Work out the finished part from the listing and answer in its coordinate system (mm). A direction names the side the tool comes from. Give positions to 0.01 mm unless a question says otherwise; leave off trailing zeros. Order: outer loops, then holes, each group sorted by start corner. A loop starts at its lowest first (then second) coordinate and runs counter-clockwise, first axis right, second up. Notation, with made-up numbers: M 86.5,-6 L 93.5,-6 A20 cw 93.5,10 Z; hole C 43.25,-25.5 d5. An arc over 180 degrees is marked long. One line per item, written item: value.
from build123d import *

# Parameters (mm, degrees)
BOSS_EXTRUDE1_DEPTH = 2
CHAMFER1_SIZE       = 12
SKETCH2_R           = 1.5
CUT_EXTRUDE1_DEPTH  = 10


with BuildPart() as part:
    # Sketch1 → Boss-Extrude1 (new body)
    with BuildSketch(Plane(origin=(0, 0, 0), x_dir=(1, 0, 0), z_dir=(0, 1, 0))):
        Polygon((-25.833763343, 95.703211573), (11.576236657, 95.703211573), (11.576236657, -6.301788427), (-25.833763343, -6.301788427), (-45.833763343, 13.698211573), (-45.833763343, 75.703211573), align=None)
        with BuildLine():
            Line((1.925471464, 43.200711573), (-28.074528536, 43.200711573))
            ThreePointArc((-28.074528536, 43.200711573), (-29.574528536, 44.700711573), (-28.074528536, 46.200711573))
            Line((-28.074528536, 46.200711573), (1.925471464, 46.200711573))
            ThreePointArc((1.925471464, 46.200711573), (3.425471464, 44.700711573), (1.925471464, 43.200711573))
        make_face(mode=Mode.SUBTRACT)
        with BuildLine():
            Line((1.925471464, 53.200711573), (-28.074528536, 53.200711573))
            ThreePointArc((-28.074528536, 53.200711573), (-29.574528536, 54.700711573), (-28.074528536, 56.200711573))
            Line((-28.074528536, 56.200711573), (1.925471464, 56.200711573))
            ThreePointArc((1.925471464, 56.200711573), (3.425471464, 54.700711573), (1.925471464, 53.200711573))
        make_face(mode=Mode.SUBTRACT)
        with BuildLine():
            Line((1.925471464, 63.200711573), (-28.074528536, 63.200711573))
            ThreePointArc((-28.074528536, 63.200711573), (-29.574528536, 64.700711573), (-28.074528536, 66.200711573))
            Line((-28.074528536, 66.200711573), (1.925471464, 66.200711573))
            ThreePointArc((1.925471464, 66.200711573), (3.425471464, 64.700711573), (1.925471464, 63.200711573))
        make_face(mode=Mode.SUBTRACT)
        with BuildLine():
            Line((1.925471464, 73.200711573), (-28.074528536, 73.200711573))
            ThreePointArc((-28.074528536, 73.200711573), (-29.574528536, 74.700711573), (-28.074528536, 76.200711573))
            Line((-28.074528536, 76.200711573), (1.925471464, 76.200711573))
            ThreePointArc((1.925471464, 76.200711573), (3.425471464, 74.700711573), (1.925471464, 73.200711573))
        make_face(mode=Mode.SUBTRACT)
        with BuildLine():
            Line((1.925471464, 83.200711573), (-28.074528536, 83.200711573))
            ThreePointArc((-28.074528536, 83.200711573), (-29.574528536, 84.700711573), (-28.074528536, 86.200711573))
            Line((-28.074528536, 86.200711573), (1.925471464, 86.200711573))
            ThreePointArc((1.925471464, 86.200711573), (3.425471464, 84.700711573), (1.925471464, 83.200711573))
        make_face(mode=Mode.SUBTRACT)
        with BuildLine():
            Line((1.925471464, 36.200711573), (-28.074528536, 36.200711573))
            ThreePointArc((-28.074528536, 36.200711573), (-29.574528536, 34.700711573), (-28.074528536, 33.200711573))
            Line((-28.074528536, 33.200711573), (1.925471464, 33.200711573))
            ThreePointArc((1.925471464, 33.200711573), (3.425471464, 34.700711573), (1.925471464, 36.200711573))
        make_face(mode=Mode.SUBTRACT)
        with BuildLine():
            Line((1.925471464, 26.200711573), (-28.074528536, 26.200711573))
            ThreePointArc((-28.074528536, 26.200711573), (-29.574528536, 24.700711573), (-28.074528536, 23.200711573))
            Line((-28.074528536, 23.200711573), (1.925471464, 23.200711573))
            ThreePointArc((1.925471464, 23.200711573), (3.425471464, 24.700711573), (1.925471464, 26.200711573))
        make_face(mode=Mode.SUBTRACT)
        with BuildLine():
            Line((1.925471464, 16.200711573), (-28.074528536, 16.200711573))
            ThreePointArc((-28.074528536, 16.200711573), (-29.574528536, 14.700711573), (-28.074528536, 13.200711573))
            Line((-28.074528536, 13.200711573), (1.925471464, 13.200711573))
            ThreePointArc((1.925471464, 13.200711573), (3.425471464, 14.700711573), (1.925471464, 16.200711573))
        make_face(mode=Mode.SUBTRACT)
        with BuildLine():
            Line((1.925471464, 6.200711573), (-28.074528536, 6.200711573))
            ThreePointArc((-28.074528536, 6.200711573), (-29.574528536, 4.700711573), (-28.074528536, 3.200711573))
            Line((-28.074528536, 3.200711573), (1.925471464, 3.200711573))
            ThreePointArc((1.925471464, 3.200711573), (3.425471464, 4.700711573), (1.925471464, 6.200711573))
        make_face(mode=Mode.SUBTRACT)
    extrude(amount=BOSS_EXTRUDE1_DEPTH)

    # Chamfer1
    chamfer1_edges = [part.edges().sort_by_distance(p)[0] for p in [
        (11.576236657, 1, -95.703211573),
        (11.576236657, 1, 6.301788427),
    ]]
    chamfer(chamfer1_edges, length=CHAMFER1_SIZE)

    # Sketch2 → Cut-Extrude1 (cut)
    with BuildSketch(Plane(origin=(0, 2, 0), x_dir=(1, 0, 0), z_dir=(0, 1, 0))):
        with Locations(Location((-4.838827122, 92.166588575, 0), (0, 0, 270))):
            Circle(SKETCH2_R)
        with Locations(Location((-41.371381926, 72.921675145, 0), (0, 0, 270))):
            Circle(SKETCH2_R)
        with Locations(Location((-41.371381926, 16.479748001, 0), (0, 0, 270))):
            Circle(SKETCH2_R)
        with Locations(Location((-4.838827122, -2.765165428, 0), (0, 0, 270))):
            Circle(SKETCH2_R)
    extrude(amount=-CUT_EXTRUDE1_DEPTH, mode=Mode.SUBTRACT)


solid = part.part
(1) Which of the six approach directions +Z, -Z, +X, -X, +Y, -Y give full straight-line access (tool end or side, diameter ignored) to faces 4 (the flat face through (-13, 1, 6.302)), 5 (the cylindrical face through (3.425, 0.986, -74.734))?
Findings:
face 4: +Z, +X, -X, +Y, -Y
face 5: +Y, -Y
(2) Determine the mould class of faces 1 (the flat face through (-13, 1, -66.201)), 2 (the flat face through (-17, 0, -57)), 3 (the flat face through (-17, 2, -57)) for opening direction Y: pulls with the +Y half, pulls with the -Y half, needs draft (parallel to the pull), parting line crosses it, or undercut.
Findings:
face 1: needs draft
face 2: pulls with the -Y half
face 3: pulls with the +Y half
(3) Find the intervals of material crossed by probe 1 along Z at (x, y) = (-40, 1.6); probe 2 along Z at (x, y) = (-41.5, 1.3); probe 3 along X at (y, z) = (0.4, -46), in increasing order. Write a range as from..to.
Findings:
probe 1: z = -81.54..-73.53, -72.31..-17.09, -15.87..-7.86
probe 2: z = -80.04..-74.42, -71.43..-17.97, -14.99..-9.36
probe 3: x = -45.83..-28.82, 2.68..11.58
(4) Section D-D, the plane z = -8.5 is taken. Give the vertices of the cut face in (x, y).
Findings:
outline: M -40.64,0 L 11.58,0 L 11.58,2 L -40.64,2 Z
(5) Given P1, Ø1, axis at x = -38.5, y = 0.5, coming from the -Z side, flat-ended and moving along its own axis, determine where the tip first touches the part or whether it passes through.
Findings:
P1: stops at z = -83.54
(6) Section B-B, the plane x = -17.5 is taken. Give the number of separate pieces and of enclosed holes in the cut face, then the cut area to 3 significant figures.
Findings:
separate pieces: 10
enclosed holes: 0
area: 150 mm^2
(7) Section A-A, the plane z = -65 is taken. Give the vertices of the cut face in (x, y), then the cut area to 3 significant figures.
Findings:
outline: M -45.83,0 L -29.54,0 L -29.54,2 L -45.83,2 Z; M 3.4,0 L 11.58,0 L 11.58,2 L 3.4,2 Z
area: 48.9 mm^2
